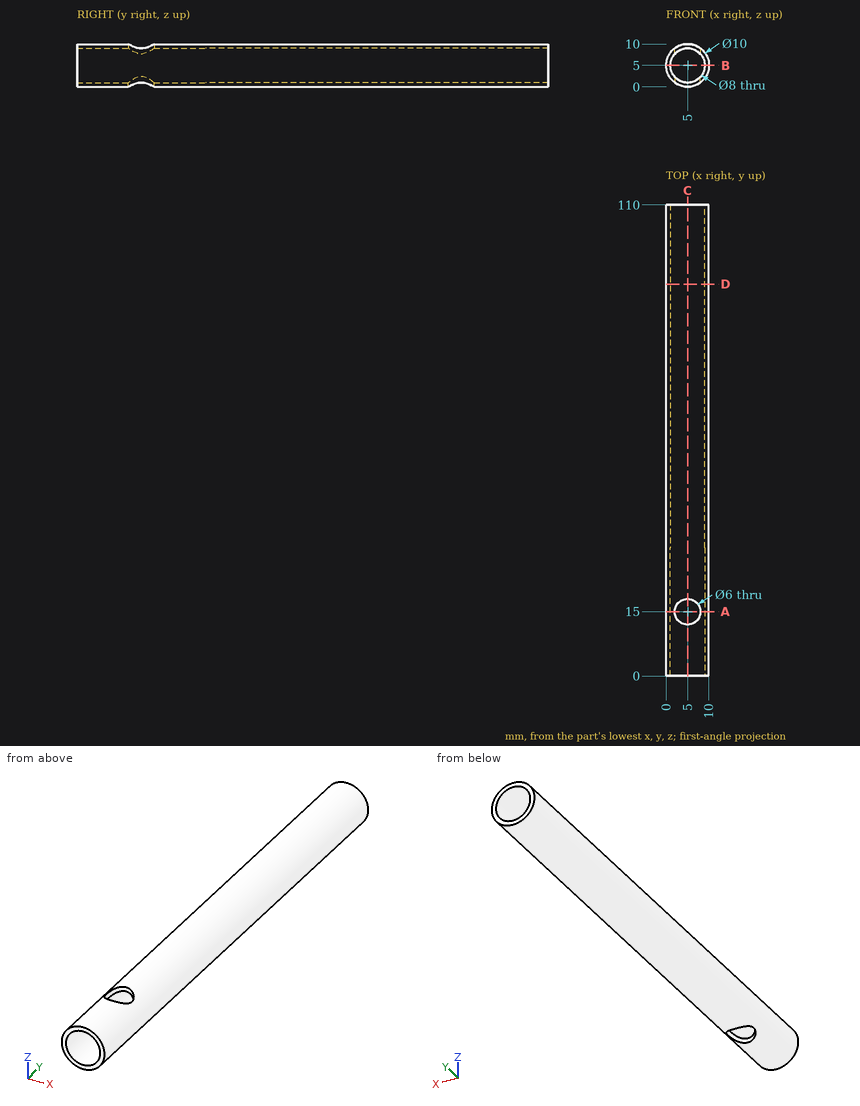
The drawing under review shows one solid part. Ordinate dimensions are in mm from its lowest x, y, z. Give positions to 0.01 mm unless a question says otherwise; leave off trailing zeros. Write each loop counter-clockwise with the first axis right and the second up, starting at its lowest first coordinate (ties: lowest second). Pieces come first, ordered by that corner, then holes. Notation, with made-up numbers: (-10, 6.5) -> (49, 6.5) arc R21 ccw to (49, 15.5) -> close; hole circle Ø1 at (-31.75, -39). An arc over 180 degrees is marked (long way). Use CSV: the item, a comma, the result in double quotes.
Q1. Take a section at C-C, the plane x = 5. Write out the cut boundary in (y, z).
Conclusion:
outline,"(0, 0) -> (12, 0) -> (12, 1) -> (0, 1) -> close; (0, 9) -> (12, 9) -> (12, 10) -> (0, 10) -> close; (18, 0) -> (110, 0) -> (110, 1) -> (18, 1) -> close; (18, 9) -> (110, 9) -> (110, 10) -> (18, 10) -> close"
Q2. Take a section at B-B, the plane z = 5. Write out the cut boundary in (x, y).
Conclusion:
outline,"(0, 0) -> (1, 0) -> (1, 110) -> (0, 110) -> close; (9, 0) -> (10, 0) -> (10, 110) -> (9, 110) -> close"
Q3. To check wall thickness, follow probe 1 along Z at (x, y) = (5, 9.5); probe 2 along X at (y, z) = (51.5, 2); probe 3 along X at (y, z) = (82, 8.5). State the ranges of each line that lie inside material, in increasing order. Write a range as [from, to].
Conclusion:
probe 1,"[0, 1], [9, 10]"
probe 2,"[1, 2.35], [7.65, 9]"
probe 3,"[1.43, 3.06], [6.94, 8.57]"
Q4. Take a section at D-D, the plane y = 91.5. Write out the cut boundary in (x, z), then the cut area to 3 significant figures.
Conclusion:
outline,"circle Ø10 at (5, 5); hole circle Ø8 at (5, 5)"
area,"28.3 mm2"
Q5. Take a section at A-A, the plane y = 15. Write out the cut boundary in (x, z), then the cut area to 3 significant figures.
Conclusion:
outline,"(2, 1) -> (2, 2.35) arc R4 cw to (2, 7.65) -> (2, 9) arc R5 ccw to start; (8, 1) arc R5 ccw to (8, 9) -> (8, 7.65) arc R4 cw to (8, 2.35) -> close"
area,"15.1 mm2"
Q6. For P1, Ø2, axis at y = 19, z = 8, coming from the -X side; P2, Ø1, axis at x = 9, y = 86.5, coming from the +Z side; P3, Ø4, axis at x = 7.5, y = 93.5, coming from the -Z side, all flat-tipped, find the tip position at first contact; note any pin that passes through.
Conclusion:
P1,"x = 0.42"
P2,"z = 8.57"
P3,"z = 0.03"
